For this review, take the finished solid that the model builds, in its own axes (mm). A direction names the side the tool comes from. Give positions to 0.01 mm unless a question says otherwise; leave off trailing zeros. Loops run counter-clockwise (first coordinate to the right, second up) from the corner with the lowest first, then second, coordinate; pieces in that order, holes last. Notation, with made-up numbers: (43, 14) - (101, 14) arc R22 cw to (101, 50) - close; hole circle Ø11 at (38, -28). An arc over 180 degrees is marked (long way). Answer in a Markdown table with one row per item.
```python
from build123d import *

# Parameters (mm, degrees)
ESQUISSE1_W                = 54
ESQUISSE1_H                = 39
BOSS_EXTRU_1_DEPTH         = 12
CONG_1_R                   = 3
CHANFREIN1_SIZE            = 0.75
ESQUISSE2_W                = 1.5
ESQUISSE2_H                = 6
ENL_V_MAT_EXTRU_1_DEPTH    = 55
ESQUISSE3_W                = 3.5
ESQUISSE3_H                = 1.5
ENL_V_MAT_EXTRU_2_DEPTH    = 55
R_P_TITION_LIN_AIRE1_COUNT = 10
R_P_TITION_LIN_AIRE1_PITCH = 3.055555556
ESQUISSE4_R                = 1.35
ENL_V_MAT_EXTRU_3_DEPTH    = 13
ENL_V_MAT_EXTRU_4_DEPTH    = 4.5


with BuildPart() as part:
    # Esquisse1 → Boss.-Extru.1 (new body)
    with BuildSketch(Plane(origin=(0, 0, 0), x_dir=(1, 0, 0), z_dir=(0, 1, 0))):
        Rectangle(ESQUISSE1_W, ESQUISSE1_H)
    extrude(amount=BOSS_EXTRU_1_DEPTH)

    # Congé1
    cong_1_edges = [part.edges().sort_by_distance(p)[0] for p in [
        (27, 6, 19.5),
        (-27, 6, 19.5),
        (-27, 6, -19.5),
        (27, 6, -19.5),
    ]]
    fillet(cong_1_edges, radius=CONG_1_R)

    # Chanfrein1
    chanfrein1_edges = [part.edges().sort_by_distance(p)[0] for p in [
        (0, 0, -19.5),
        (0, 12, -19.5),
        (27, 0, 0),
        (0, 0, 19.5),
        (-27, 0, 0),
        (-26.121320344, 0, 18.621320344),
        (-26.121320344, 0, -18.621320344),
        (26.121320344, 0, 18.621320344),
        (26.121320344, 0, -18.621320344),
        (27, 12, 0),
        (-27, 12, 0),
        (0, 12, 19.5),
        (-26.121320344, 12, 18.621320344),
        (-26.121320344, 12, -18.621320344),
        (26.121320344, 12, 18.621320344),
        (26.121320344, 12, -18.621320344),
    ]]
    chamfer(chanfrein1_edges, length=CHANFREIN1_SIZE)

    # Esquisse2 → Enlèv. mat.-Extru.1 (cut, through all)
    with BuildSketch(Plane.ZY.offset(27)):
        with Locations((-13.75, 9)):
            Rectangle(ESQUISSE2_W, ESQUISSE2_H)
    enl_v_mat_extru_1 = extrude(amount=-ENL_V_MAT_EXTRU_1_DEPTH, mode=Mode.SUBTRACT)

    # Esquisse3 → Enlèv. mat.-Extru.2 (cut, through all)
    with BuildSketch(Plane.ZY.offset(27)):
        with Locations((-17.75, 9.75)):
            Rectangle(ESQUISSE3_W, ESQUISSE3_H)
        with Locations((-17.75, 6.75)):
            Rectangle(ESQUISSE3_W, ESQUISSE3_H)
        with Locations((-17.75, 3.75)):
            Rectangle(ESQUISSE3_W, ESQUISSE3_H)
    enl_v_mat_extru_2 = extrude(amount=-ENL_V_MAT_EXTRU_2_DEPTH, mode=Mode.SUBTRACT)

    # Symétrie1: Enlèv. mat.-Extru.1, Enlèv. mat.-Extru.2 across plane
    add(enl_v_mat_extru_1.mirror(Plane.XY), mode=Mode.SUBTRACT)
    add(enl_v_mat_extru_2.mirror(Plane.XY), mode=Mode.SUBTRACT)

    # Répétition linéaire1: Enlèv. mat.-Extru.1 ×10
    with Locations(*[(0, 0, i * R_P_TITION_LIN_AIRE1_PITCH) for i in range(1, R_P_TITION_LIN_AIRE1_COUNT)]):
        add(enl_v_mat_extru_1, mode=Mode.SUBTRACT)

    # Esquisse4 → Enlèv. mat.-Extru.3 (cut, through all)
    with BuildSketch(Plane(origin=(0, 12, 0), x_dir=(1, 0, 0), z_dir=(0, 1, 0))):
        with Locations(Location((-24, 16.5, 0), (0, 0, 270))):  # turned: the seam where the file's is
            Circle(ESQUISSE4_R)
        with Locations(Location((24, 16.5, 0), (0, 0, 270))):  # turned: the seam where the file's is
            Circle(ESQUISSE4_R)
        with Locations(Location((24, -16.5, 0), (0, 0, 270))):  # turned: the seam where the file's is
            Circle(ESQUISSE4_R)
        with Locations(Location((-24, -16.5, 0), (0, 0, 270))):  # turned: the seam where the file's is
            Circle(ESQUISSE4_R)
    extrude(amount=-ENL_V_MAT_EXTRU_3_DEPTH, mode=Mode.SUBTRACT)

    # Esquisse5 → Enlèv. mat.-Extru.4 (cut)
    with BuildSketch(Plane.XZ):
        with BuildLine():
            Line((-24, 13.5), (-27, 13.5))
            Line((-27, 13.5), (-27, -13.5))
            Line((-27, -13.5), (-24, -13.5))
            ThreePointArc((-24, -13.5), (-21.878679656, -14.378679656), (-21, -16.5))
            Line((-21, -16.5), (-21, -19.5))
            Line((-21, -19.5), (21, -19.5))
            Line((21, -19.5), (21, -16.5))
            ThreePointArc((21, -16.5), (21.878679656, -14.378679656), (24, -13.5))
            Line((24, -13.5), (27, -13.5))
            Line((27, -13.5), (27, 13.5))
            Line((27, 13.5), (24, 13.5))
            ThreePointArc((24, 13.5), (21.878679656, 14.378679656), (21, 16.5))
            Line((21, 16.5), (21, 19.5))
            Line((21, 19.5), (-21, 19.5))
            Line((-21, 19.5), (-21, 16.5))
            ThreePointArc((-21, 16.5), (-21.878679656, 14.378679656), (-24, 13.5))
        make_face()
    extrude(amount=-ENL_V_MAT_EXTRU_4_DEPTH, mode=Mode.SUBTRACT)


solid = part.part
```
1. Clearance check with flat-ended pins moving along their axes: pin 1 (2.5 mm diameter, centred on x = 26, y = 2.5, fed in from -Z); pin 2 (1.6 mm diameter, centred on x = 3.5, z = 14, fed in from +Y); pin 3 (2 mm diameter, centred on x = 5.5, z = 0.5, fed in from -Y); pin 4 (0.8 mm diameter, centred on x = 6.5, z = 11, fed in from +Y). State where each tip first meets the part, or that it passes through.
Values:
| item | result |
|---|---|
| pin 1 | stops at z = -19.4 |
| pin 2 | stops at y = 12 |
| pin 3 | stops at y = 4.5 |
| pin 4 | stops at y = 6 |
2. Wall thickness on line 1 (Y direction, x = -10, z = -17); line 2 (Y direction, x = 20, z = -2); line 3 (Y direction, x = -23, z = 6): over which ranges is each line inside the solid? List them lowest first. Write a range as [from, to].
Values:
| item | result |
|---|---|
| line 1 | y = [4.5, 6], [7.5, 9], [10.5, 12] |
| line 2 | y = [4.5, 6] |
| line 3 | y = [4.5, 12] |
3. For faces 5 (the face through (0, 6, 18)), 6 (the face through (0, 6, -18)), 7 (the face through (0, 6, 8)), list the 3-axis set-ups (+Z, -Z, +X, -X, +Y, -Y) from which the entire face can be reached by the end or side of a thin tool; tool diameter is ignored.
Values:
| item | result |
|---|---|
| face 5 | +Z, +X, -X |
| face 6 | -Z, +X, -X |
| face 7 | +X, -X, +Y |
4. Mouldability with a two-part tool opening along X and no side actions: class faces 1 (the face through (-26.14, 10.88, -18.6)), 2 (the face through (-23.594, 6.084, -15.212)), 3 (the face through (0, 8, -19.5)), 4 (the face through (25.76, 11.79, 18.22)) as released by +X, released by -X, zero draft, split by the parting line, or undercut.
Values:
| item | result |
|---|---|
| face 1 | released by -X |
| face 2 | undercut |
| face 3 | zero draft |
| face 4 | released by +X |
5. We need section B-B, the plane z = 4.5. Give the boundary of the cut face in (x, y), and give its area (3 significant figures).
Values:
| item | result |
|---|---|
| outline | (-27, 4.5) - (27, 4.5) - (27, 6) - (-27, 6) - close |
| area | 81.0 mm^2 |
6. We need section A-A, the plane y = 2. Give the boundary of the cut face in (x, z), and give its area (3 significant figures).
Values:
| item | result |
|---|---|
| outline | (-27, -16.5) arc R3 ccw to (-24, -19.5) - (-21, -19.5) - (-21, -16.5) arc R3 ccw to (-24, -13.5) - (-27, -13.5) - close; (-27, 13.5) - (-24, 13.5) arc R3 ccw to (-21, 16.5) - (-21, 19.5) - (-24, 19.5) arc R3 ccw to (-27, 16.5) - close; (21, -19.5) - (24, -19.5) arc R3 ccw to (27, -16.5) - (27, -13.5) - (24, -13.5) arc R3 ccw to (21, -16.5) - close; (21, 16.5) arc R3 ccw to (24, 13.5) - (27, 13.5) - (27, 16.5) arc R3 ccw to (24, 19.5) - (21, 19.5) - close; hole circle Ø2.7 at (-24, -16.5); hole circle Ø2.7 at (-24, 16.5); hole circle Ø2.7 at (24, -16.5); hole circle Ø2.7 at (24, 16.5) |
| area | 106 mm^2 |
